Here's how the part is built. I have some questions about the finished solid (model axes, mm). A direction names the side the tool comes from. Coordinates: 2 decimals unless noted, no trailing zeros. Order: outer loops, then holes, each group sorted by start corner. A loop starts at its lowest first (then second) coordinate and runs counter-clockwise, first axis right, second up. Notation, with made-up numbers: (37.5, 44.25) - (90.5, 44.25) arc R22 ccw to (90.5, 53.25) - close; hole circle Ø6 at (-36, 22.25). An arc over 180 degrees is marked (long way). Answer as CSV lines item,"result". Start each with the question number.
Q1. For faces 1 (the face through (22, 24, 5)), 2 (the face through (40, 72, -2)), 3 (the face through (15, 72, 0)), which set-ups out of +Z, -Z, +X, -X, +Y, -Y let a thin tool reach every point of the face, with its end or its side?
Q2. I need wall thicknesses on line 1 (X direction, y = 112, z = 2.5); line 2 (Y direction, x = 25.5, z = 6); line 3 (X direction, y = 115.5, z = 5.25). Which ranges of each line are inside material? Lowest first, please.
Q3. For pin 1 Ø0.6 at (y, z) = (23, -3.5) entering from -X; pin 2 Ø1.5 at (x, y) = (22.5, 23.5) entering from +Z; pin 3 Ø4 at (x, y) = (22.5, 117.5) entering from -Z, each with a flat end and sliding along its axis, tell me the tip position at first contact or that it passes through.
Q4. Suppose I cut it at C-C (z = 1.75). Please give me the cut outline in (x, y), then the cut area to 4 significant figures.
Q5. Suppose I cut it at A-A (y = 76.5). Please give me the cut outline in (x, z), then the cut area to 3 significant figures.
Q6. Suppose I cut it at B-B (x = 18). Please give me the cut outline in (y, z), then the cut area to 3 significant figures.
Q7. Suppose I cut it at D-D (x = 38). Please give me the cut outline in (y, z).
Q8. Thinking about a two-plate mould opening in Y: for faces 4 (the face through (22, 131, 3)), 5 (the face through (2, 66, 0)), 6 (the face through (22.3, 21, -1.5)), 7 (the face through (5, 70, 5)), which applies, released by +Y, released by -Y, zero draft, split by the parting line, or undercut?
from build123d import *

# Parameters (mm, degrees)
F0_W      = 45
F0_H      = 131
F1_DEPTH  = 2
F2_W      = 45
F2_H      = 131
F3_DEPTH  = 5
F5_W      = 35
F5_H      = 100
F6_DEPTH  = 4
F7_W      = 5
F7_H      = 100
F8_DEPTH  = 2
F4_W      = 15
F4_H      = 90
F9_DEPTH  = 7.001
F10_W     = 5
F10_H     = 5
F13_DEPTH = 2
F12_W     = 5
F12_H     = 5
F14_DEPTH = 4
F11_W     = 10
F11_H     = 100
F15_DEPTH = 4


with BuildPart() as f1:
    # F0 (on Top) → F1 (new body)
    with BuildSketch(Plane.XY):
        with Locations((22.5, 65.5)):
            Rectangle(F0_W, F0_H)
    extrude(amount=F1_DEPTH)

    # F2 (on face) → F3 (join)
    with BuildSketch(Plane.XY.offset(2)):
        with Locations((22.5, 65.5)):
            Rectangle(F2_W, F2_H)
    extrude(amount=F3_DEPTH)

    # F5 (on face) → F6 (cut)
    with BuildSketch(Plane.XY.offset(7)):
        with Locations((22.5, 71)):
            Rectangle(F5_W, F5_H)
    extrude(amount=-F6_DEPTH, mode=Mode.SUBTRACT)

    # F7 (on face) → F8 (join)
    with BuildSketch(Plane.XY.offset(3)):
        with Locations((22.5, 71)):
            Rectangle(F7_W, F7_H)
    extrude(amount=F8_DEPTH)

    # F4 (on face) → F9 (cut, through all)
    with BuildSketch(Plane.XY.offset(7)):
        with Locations((22.5, 71)):
            Rectangle(F4_W, F4_H)
    extrude(amount=-F9_DEPTH, mode=Mode.SUBTRACT)

    # F10 (on face) → F13 (join)
    with BuildSketch(Plane(origin=(0, 0, 0), x_dir=(1, 0, 0), z_dir=(0, 0, -1))):
        with Locations((22.5, -118.5)):
            Rectangle(F10_W, F10_H)
        with Locations((22.5, -23.5)):
            Rectangle(F10_W, F10_H)
    extrude(amount=F13_DEPTH)

    # F12 (on face) → F14 (join)
    with BuildSketch(Plane(origin=(0, 0, 0), x_dir=(1, 0, 0), z_dir=(0, 0, -1))):
        with Locations((17.5, -23.5)):
            Rectangle(F12_W, F12_H)
        with Locations((27.5, -23.5)):
            Rectangle(F12_W, F12_H)
        with Locations((27.5, -118.5)):
            Rectangle(F12_W, F12_H)
        with Locations((17.5, -118.5)):
            Rectangle(F12_W, F12_H)
    extrude(amount=F14_DEPTH)

    # F11 (on face) → F15 (join)
    with BuildSketch(Plane(origin=(0, 0, 0), x_dir=(1, 0, 0), z_dir=(0, 0, -1))):
        with Locations((10, -71)):
            Rectangle(F11_W, F11_H)
        with Locations((35, -71)):
            Rectangle(F11_W, F11_H)
    extrude(amount=F15_DEPTH)


solid = f1.part
Here are the results:
1,face 1,"+Z"
1,face 2,"-Z, +X, +Y, -Y"
1,face 3,"+Z, -Z"
2,line 1,"x = 0 to 15, 30 to 45"
2,line 2,"y = 0 to 21, 121 to 131"
2,line 3,"x = 0 to 5, 40 to 45"
3,pin 1,"stops at x = 5"
3,pin 2,"stops at z = 5"
3,pin 3,"stops at z = -2"
4,outline,"(0, 0) - (45, 0) - (45, 131) - (0, 131) - close; hole (15, 26) - (30, 26) - (30, 116) - (15, 116) - close"
4,area,"4,545 mm²"
5,outline,"(0, 0) - (5, 0) - (5, -4) - (15, -4) - (15, 3) - (5, 3) - (5, 7) - (0, 7) - close; (30, -4) - (40, -4) - (40, 0) - (45, 0) - (45, 7) - (40, 7) - (40, 3) - (30, 3) - close"
5,area,"210 mm²"
6,outline,"(0, 0) - (21, 0) - (21, -4) - (26, -4) - (26, 3) - (21, 3) - (21, 7) - (0, 7) - close; (116, -4) - (121, -4) - (121, 0) - (131, 0) - (131, 7) - (121, 7) - (121, 3) - (116, 3) - close"
6,area,"287 mm²"
7,outline,"(0, 0) - (21, 0) - (21, -4) - (121, -4) - (121, 0) - (131, 0) - (131, 7) - (121, 7) - (121, 3) - (21, 3) - (21, 7) - (0, 7) - close"
8,face 4,"released by +Y"
8,face 5,"zero draft"
8,face 6,"released by -Y"
8,face 7,"undercut"
